Design review of the part built by this model. Coordinates are the model's own, in mm. A direction names the side the tool comes from. Coordinates: 2 decimals unless noted, no trailing zeros. Order: outer loops, then holes, each group sorted by start corner. A loop starts at its lowest first (then second) coordinate and runs counter-clockwise, first axis right, second up. Notation, with made-up numbers: M 46.25,14.25 L 98.25,14.25 A23 ccw 98.25,43.25 Z; hole C 58,83 d2. An arc over 180 degrees is marked long. Answer as a JSON object with one key per item and string values.
from build123d import *

# Parameters (mm, degrees)
SKETCH1_W           = 25.4
SKETCH1_H           = 25.4
SKETCH1_W_2         = 19.05
SKETCH1_H_2         = 19.05
BOSS_EXTRUDE1_DEPTH = 488.95
CUT_EXTRUDE1_REACH  = 492.268
SKETCH2_R           = 1.7
SKETCH5_W           = 19.05
SKETCH5_H           = 25.400569513
CUT_EXTRUDE2_DEPTH  = 491.267704933
CUT_EXTRUDE3_REACH  = 492.268
SKETCH6_R           = 3.2639


with BuildPart() as part:
    # Sketch1 → Boss-Extrude1 (new body)
    with BuildSketch(Plane(origin=(0, 0, 0), x_dir=(1, 0, 0), z_dir=(0, 1, 0))):
        with Locations((12.7, -12.7)):
            Rectangle(SKETCH1_W, SKETCH1_H)
        with Locations((12.7, -12.7)):
            Rectangle(SKETCH1_W_2, SKETCH1_H_2, mode=Mode.SUBTRACT)
    extrude(amount=BOSS_EXTRUDE1_DEPTH)

    # Cut-Extrude1: up to this face of the body (flat: up to its plane)
    cut_extrude1_end = Plane(part.part.faces().sort_by_distance((12.7, 244.475, 25.4))[0])
    # Sketch2 → Cut-Extrude1 (cut, up to the picked face)
    with BuildSketch(Plane(origin=(0, 0, 0), x_dir=(-1, 0, 0), z_dir=(0, 0, -1)), mode=Mode.PRIVATE) as cut_extrude1_sk1:
        with Locations((-5.7, 232.350644347)):
            Circle(SKETCH2_R)
    cut_extrude1_tool1 = split(extrude(cut_extrude1_sk1.sketch, amount=-CUT_EXTRUDE1_REACH, mode=Mode.PRIVATE), bisect_by=cut_extrude1_end, keep=Keep.BOTH, mode=Mode.PRIVATE)
    # Sketch2 → Cut-Extrude1 (cut, up to the picked face)
    with BuildSketch(Plane(origin=(0, 0, 0), x_dir=(-1, 0, 0), z_dir=(0, 0, -1)), mode=Mode.PRIVATE) as cut_extrude1_sk2:
        with Locations((-19.7, 232.350644347)):
            Circle(SKETCH2_R)
    cut_extrude1_tool2 = split(extrude(cut_extrude1_sk2.sketch, amount=-CUT_EXTRUDE1_REACH, mode=Mode.PRIVATE), bisect_by=cut_extrude1_end, keep=Keep.BOTH, mode=Mode.PRIVATE)
    # Sketch2 → Cut-Extrude1 (cut, up to the picked face)
    with BuildSketch(Plane(origin=(0, 0, 0), x_dir=(-1, 0, 0), z_dir=(0, 0, -1)), mode=Mode.PRIVATE) as cut_extrude1_sk3:
        with Locations((-19.7, 256.599355653)):
            Circle(SKETCH2_R)
    cut_extrude1_tool3 = split(extrude(cut_extrude1_sk3.sketch, amount=-CUT_EXTRUDE1_REACH, mode=Mode.PRIVATE), bisect_by=cut_extrude1_end, keep=Keep.BOTH, mode=Mode.PRIVATE)
    # Sketch2 → Cut-Extrude1 (cut, up to the picked face)
    with BuildSketch(Plane(origin=(0, 0, 0), x_dir=(-1, 0, 0), z_dir=(0, 0, -1)), mode=Mode.PRIVATE) as cut_extrude1_sk4:
        with Locations((-5.7, 256.599355653)):
            Circle(SKETCH2_R)
    cut_extrude1_tool4 = split(extrude(cut_extrude1_sk4.sketch, amount=-CUT_EXTRUDE1_REACH, mode=Mode.PRIVATE), bisect_by=cut_extrude1_end, keep=Keep.BOTH, mode=Mode.PRIVATE)
    add(cut_extrude1_tool1.solids().sort_by(Axis((5.7, 232.350644, 0), (0, 0, 1)))[0], mode=Mode.SUBTRACT)
    add(cut_extrude1_tool2.solids().sort_by(Axis((19.7, 232.350644, 0), (0, 0, 1)))[0], mode=Mode.SUBTRACT)
    add(cut_extrude1_tool3.solids().sort_by(Axis((19.7, 256.599356, 0), (0, 0, 1)))[0], mode=Mode.SUBTRACT)
    add(cut_extrude1_tool4.solids().sort_by(Axis((5.7, 256.599356, 0), (0, 0, 1)))[0], mode=Mode.SUBTRACT)

    # Sketch5 → Cut-Extrude2 (cut, through all)
    with BuildSketch(Plane.ZY):
        with Locations((12.7, 12.700284757)):
            Rectangle(SKETCH5_W, SKETCH5_H)
    cut_extrude2 = extrude(amount=-CUT_EXTRUDE2_DEPTH, mode=Mode.SUBTRACT)

    # Mirror1: Cut-Extrude2 across plane
    add(cut_extrude2.mirror(Plane.ZX.offset(244.475)), mode=Mode.SUBTRACT)

    # Cut-Extrude3: up to this face of the body (flat: up to its plane)
    cut_extrude3_end = Plane(part.part.faces().sort_by_distance((12.7, 244.475, 0))[0])
    # Sketch6 → Cut-Extrude3 (cut, up to the picked face)
    with BuildSketch(Plane.XY.offset(25.4), mode=Mode.PRIVATE) as cut_extrude3_sk1:
        with Locations((12.7, 12.7)):
            Circle(SKETCH6_R)
    cut_extrude3_tool1 = split(extrude(cut_extrude3_sk1.sketch, amount=-CUT_EXTRUDE3_REACH, mode=Mode.PRIVATE), bisect_by=cut_extrude3_end, keep=Keep.BOTH, mode=Mode.PRIVATE)
    cut_extrude3 = cut_extrude3_tool1.solids().sort_by(Axis((12.7, 12.7, 25.4), (0, 0, -1)))[0]
    add(cut_extrude3, mode=Mode.SUBTRACT)

    # Mirror2: Cut-Extrude3 across plane
    add(cut_extrude3.mirror(Plane.ZX.offset(244.475)), mode=Mode.SUBTRACT)


solid = part.part
1) Add section B-B (z = 14.5). State the section outline as (x, y) points (3 decimals).
Taken from the geometry:
{"outline": "M 0,25.401 L 3.175,25.401 L 3.175,463.549 L 0,463.549 Z; M 22.225,25.401 L 25.4,25.401 L 25.4,463.549 L 22.225,463.549 Z"}
2) To check wall thickness, follow L1, parallel to Y at x = 5.7, z = 22.9; L2, parallel to Z at x = 8, y = 126 (3 decimals). State the ranges of each line that lie inside material, in increasing order.
Taken from the geometry:
{"L1": "y = 0 to 230.65, 234.05 to 254.9, 258.3 to 488.95", "L2": "z = 0 to 3.175, 22.225 to 25.4"}
3) Insertion check: pin 1 Ø1.6 at (x, z) = (2, 10.5) entering from -Y; pin 2 Ø2 at (x, y) = (5.7, 232.35) entering from +Z; pin 3 Ø3.5 at (x, z) = (1.5, 13.5) entering from +Y. Each pin has a flat end and moves straight along its axis. Give the tip position at first contact, or say it passes through.
Taken from the geometry:
{"pin 1": "stops at y = 25.4", "pin 2": "passes through", "pin 3": "stops at y = 463.55"}
4) Tool access review of faces 1 (the flat face through (3.175, 241, 13)), 2 (the flat face through (25.4, 241, 13)): name each direction out of +Z, -Z, +X, -X, +Y, -Y from which nothing blocks a thin tool from reaching the whole face with its end or side.
Taken from the geometry:
{"face 1": "+Y, -Y", "face 2": "+Z, -Z, +X, +Y, -Y"}
5) Mouldability with a two-part tool opening along Z and no side actions: class faces 3 (the flat face through (13, 241, 25.4)), 4 (the flat face through (22.225, 241, 13)), 5 (the flat face through (13, 241, 0)) as released by +Z, released by -Z, zero draft, split by the parting line, or undercut.
Taken from the geometry:
{"face 3": "released by +Z", "face 4": "undercut", "face 5": "released by -Z"}
6) Add section A-A (y = 196.5). State the section outline as (x, z) points (3 decimals).
Taken from the geometry:
{"outline": "M 0,0 L 25.4,0 L 25.4,25.4 L 0,25.4 Z; hole M 3.175,3.175 L 22.225,3.175 L 22.225,22.225 L 3.175,22.225 Z"}
